Could you check a few things on this model? Use its own coordinates, in mm. Face numbers are marked on the shaded views. A direction names the side the tool comes from. Round coordinates to 2 decimals unless told otherwise and drop trailing zeros. Loops run counter-clockwise (first coordinate to the right, second up) from the corner with the lowest first, then second, coordinate; pieces in that order, holes last.
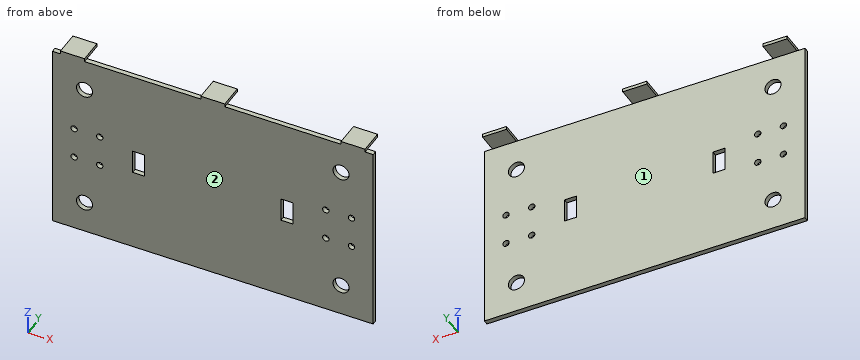
from build123d import *

# Parameters (mm, degrees)
SKETCH1_W           = 200
SKETCH1_H           = 120
BOSS_EXTRUDE3_DEPTH = 1
SKETCH3_W           = 200
SKETCH3_H           = 120
SKETCH3_R           = 5
BOSS_EXTRUDE4_DEPTH = 2
SKETCH10_W          = 15
SKETCH10_H          = 15
BOSS_EXTRUDE6_DEPTH = 2
SKETCH12_R          = 2
SKETCH12_W          = 7.5
SKETCH12_H          = 15
CUT_EXTRUDE1_DEPTH  = 119.612815496
CUT_EXTRUDE2_START  = -10
SKETCH8_R           = 5
CUT_EXTRUDE2_DEPTH  = 10


with BuildPart() as part:
    # Sketch1 → Boss-Extrude3 (new body)
    with BuildSketch(Plane(origin=(0, 0, 0), x_dir=(1, 0, 0), z_dir=(0, 1, 0))):
        Rectangle(SKETCH1_W, SKETCH1_H)
    extrude(amount=BOSS_EXTRUDE3_DEPTH)

    # Sketch3 → Boss-Extrude4 (add)
    # profile 1 of 4: a face of its own
    with BuildSketch(Plane(origin=(0, 1, 0), x_dir=(1, 0, 0), z_dir=(0, 1, 0))):
        Rectangle(SKETCH3_W, SKETCH3_H)
        with Locations(Location((-80, -40, 0), (0, 0, 270))):
            Circle(SKETCH3_R, mode=Mode.SUBTRACT)
        with Locations(Location((80, -40, 0), (0, 0, 270))):
            Circle(SKETCH3_R, mode=Mode.SUBTRACT)
        with Locations(Location((-80, 40, 0), (0, 0, 270))):
            Circle(SKETCH3_R, mode=Mode.SUBTRACT)
        with Locations(Location((80, 40, 0), (0, 0, 270))):
            Circle(SKETCH3_R, mode=Mode.SUBTRACT)
    # profile 2 of 4: a face of its own
    with BuildSketch(Plane(origin=(0, 1, 0), x_dir=(1, 0, 0), z_dir=(0, 1, 0))):
        Rectangle(SKETCH3_W, SKETCH3_H)
        with Locations(Location((-80, -40, 0), (0, 0, 270))):
            Circle(SKETCH3_R, mode=Mode.SUBTRACT)
        with Locations(Location((80, -40, 0), (0, 0, 270))):
            Circle(SKETCH3_R, mode=Mode.SUBTRACT)
        with Locations(Location((-80, 40, 0), (0, 0, 270))):
            Circle(SKETCH3_R, mode=Mode.SUBTRACT)
        with Locations(Location((80, 40, 0), (0, 0, 270))):
            Circle(SKETCH3_R, mode=Mode.SUBTRACT)
    # profile 3 of 4: a face of its own
    with BuildSketch(Plane(origin=(0, 1, 0), x_dir=(1, 0, 0), z_dir=(0, 1, 0))):
        Rectangle(SKETCH3_W, SKETCH3_H)
        with Locations(Location((-80, -40, 0), (0, 0, 270))):
            Circle(SKETCH3_R, mode=Mode.SUBTRACT)
        with Locations(Location((80, -40, 0), (0, 0, 270))):
            Circle(SKETCH3_R, mode=Mode.SUBTRACT)
        with Locations(Location((-80, 40, 0), (0, 0, 270))):
            Circle(SKETCH3_R, mode=Mode.SUBTRACT)
        with Locations(Location((80, 40, 0), (0, 0, 270))):
            Circle(SKETCH3_R, mode=Mode.SUBTRACT)
    # profile 4 of 4: a face of its own
    with BuildSketch(Plane(origin=(0, 1, 0), x_dir=(1, 0, 0), z_dir=(0, 1, 0))):
        Rectangle(SKETCH3_W, SKETCH3_H)
        with Locations(Location((-80, -40, 0), (0, 0, 270))):
            Circle(SKETCH3_R, mode=Mode.SUBTRACT)
        with Locations(Location((80, -40, 0), (0, 0, 270))):
            Circle(SKETCH3_R, mode=Mode.SUBTRACT)
        with Locations(Location((-80, 40, 0), (0, 0, 270))):
            Circle(SKETCH3_R, mode=Mode.SUBTRACT)
        with Locations(Location((80, 40, 0), (0, 0, 270))):
            Circle(SKETCH3_R, mode=Mode.SUBTRACT)
    extrude(amount=BOSS_EXTRUDE4_DEPTH)

    # Sketch10 → Boss-Extrude6 (add)
    with BuildSketch(Plane.XY.offset(60)):
        with Locations((-87.5, 7.5)):
            Rectangle(SKETCH10_W, SKETCH10_H)
        with Locations((87.5, 7.5)):
            Rectangle(SKETCH10_W, SKETCH10_H)
        with Locations((0, 7.5)):
            Rectangle(SKETCH10_W, SKETCH10_H)
    extrude(amount=BOSS_EXTRUDE6_DEPTH)

    # Sketch12 → Cut-Extrude1 (cut, through all)
    with BuildSketch(Plane.XZ):
        with Locations(Location((-86.5, 10, 0), (0, 0, 270))):
            Circle(SKETCH12_R)
        with Locations(Location((-70.5, 10, 0), (0, 0, 270))):
            Circle(SKETCH12_R)
        with Locations(Location((-70.5, -10, 0), (0, 0, 90))):
            Circle(SKETCH12_R)
        with Locations(Location((-86.5, -10, 0), (0, 0, 90))):
            Circle(SKETCH12_R)
        with Locations(Location((86.5, -10, 0), (0, 0, 270))):
            Circle(SKETCH12_R)
        with Locations(Location((70.5, -10, 0), (0, 0, 270))):
            Circle(SKETCH12_R)
        with Locations(Location((70.5, 10, 0), (0, 0, 90))):
            Circle(SKETCH12_R)
        with Locations(Location((86.5, 10, 0), (0, 0, 90))):
            Circle(SKETCH12_R)
        with Locations((46.25, 0)):
            Rectangle(SKETCH12_W, SKETCH12_H)
        with Locations((-46.25, 0)):
            Rectangle(SKETCH12_W, SKETCH12_H)
    extrude(amount=-CUT_EXTRUDE1_DEPTH, mode=Mode.SUBTRACT)

    # Sketch8 → Cut-Extrude2 (cut)
    with BuildSketch(Plane(origin=(0, 3, 0), x_dir=(1, 0, 0), z_dir=(0, 1, 0)).offset(CUT_EXTRUDE2_START)):
        with Locations(Location((-80, 40, 0), (0, 0, 270))):
            Circle(SKETCH8_R)
        with Locations(Location((80, 40, 0), (0, 0, 270))):
            Circle(SKETCH8_R)
        with Locations(Location((80, -40, 0), (0, 0, 270))):
            Circle(SKETCH8_R)
        with Locations(Location((-80, -40, 0), (0, 0, 270))):
            Circle(SKETCH8_R)
    extrude(amount=CUT_EXTRUDE2_DEPTH, mode=Mode.SUBTRACT)


solid = part.part
Item 1: Will these pins go through, and if not, where does the flat tip stop? pin 1 (3 mm diameter, centred on x = -65.5, z = -21, fed in from +Y); pin 2 (5 mm diameter, centred on x = 73, y = 4.5, fed in from +Z); pin 3 (2 mm diameter, centred on y = 10.5, z = 61.5, fed in from -X).
Results list:
pin 1: stops at y = 3
pin 2: stops at z = 60
pin 3: stops at x = -95
Item 2: If we section it at B-B, the plane x = -70.5: Please give me the cut outline in (y, z), then the cut area to 3 significant figures.
Results list:
outline: (0, -60) - (3, -60) - (3, -12) - (0, -12) - close; (0, -8) - (3, -8) - (3, 8) - (0, 8) - close; (0, 12) - (3, 12) - (3, 60) - (0, 60) - close
area: 336 mm2
Item 3: If I drill on line 1 along X through (y, z) = (2.1, 40); line 2 along X through (y, z) = (1.25, 10); line 3 along Y through (x, z) = (-59.5, 20), over which ranges is the centre line in solid material (lowest first)?
Results list:
line 1: x = -100 to -85, -75 to 75, 85 to 100
line 2: x = -100 to -88.5, -84.5 to -72.5, -68.5 to 68.5, 72.5 to 84.5, 88.5 to 100
line 3: y = 0 to 3
Item 4: If we section it at A-A, the plane z = -1: Please give me the cut outline in (x, y), then the cut area to 3 significant figures.
Results list:
outline: (-100, 0) - (-50, 0) - (-50, 3) - (-100, 3) - close; (-42.5, 0) - (42.5, 0) - (42.5, 3) - (-42.5, 3) - close; (50, 0) - (100, 0) - (100, 3) - (50, 3) - close
area: 555 mm2
Item 5: If we section it at C-C, the plane x = 0: Please give me the cut outline in (y, z), then the cut area to 3 significant figures.
Results list:
outline: (0, -60) - (3, -60) - (3, 60) - (15, 60) - (15, 62) - (0, 62) - close
area: 390 mm2
Item 6: If we section it at D-D, the plane z = 30: Please give me the cut outline in (x, y), then the cut area to 3 significant figures.
Results list:
outline: (-100, 0) - (100, 0) - (100, 3) - (-100, 3) - close
area: 600 mm2
Item 7: For the marked faces 1 and 2, which set-ups out of +Z, -Z, +X, -X, +Y, -Y let a thin tool reach every point of the face, with its end or its side?
Results list:
face 1: -Z, +X, -X, +Y
face 2: +Z, -Z, +X, -X, -Y
